Solid Edge part; units mm, degrees
sketch "Sketch1" plane through (0, 0, 0) normal (0, 0, 1) x (1, 0, 0)
  line L0 (0, 0) -> (-248.03, 0)
  line L1 (-248.03, 0) -> (-248.03, -85)
  line L2 (-248.03, -85) -> (0, -85)
  line L3 (0, -85) -> (0, 0)
extrude "Protrusion1" add sketch "Sketch1" against normal blind 20.4
sketch "Sketch2" plane through (-124.015, -42.5, 0) normal (0, 0, 1) x (1, 0, 0)
  circle A0 centre (155, -6) radius 55
  circle A1 centre (57.5, -9) radius 6.7
extrude "ExtrudedCutout_1" cut sketch "Sketch2" against normal blind 20.5
chamfer "Chamfer_2" distance 2 angle 45 1 edges at (-10.158, -85, -10.2)
fillet "Round_1" radius 1 1 edges at (0, 0, -10.2)
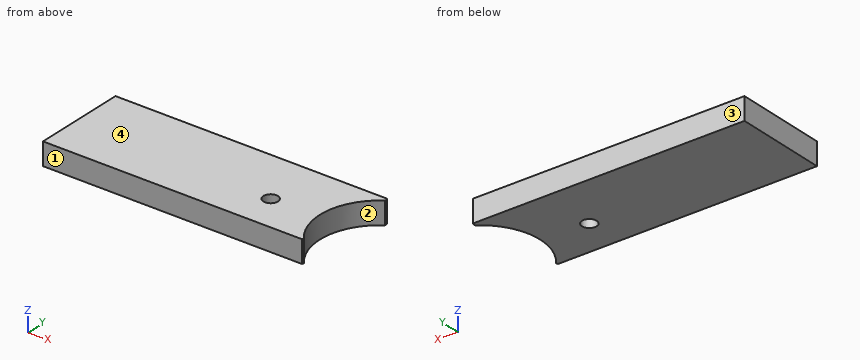
Design review of the part built by this model. Coordinates are the model's own, in mm. Face numbers are marked on the shaded views. Coordinates: 2 decimals unless noted, no trailing zeros. Order: outer loops, then holes, each group sorted by start corner. A loop starts at its lowest first (then second) coordinate and runs counter-clockwise, first axis right, second up. Notation, with made-up numbers: (-34, 14.25) -> (-8, 14.25) arc R21 cw to (-8, 53.25) -> close; hole circle Ø8 at (86.5, 24.5). An arc over 180 degrees is marked (long way). Use one line per item in the form item = value. Start each with the question number.
(1) Insertion check: pin 1 (8 mm diameter, centred on x = -66.515, y = -51.5, fed in from -Z). The pin has a flat end and moves straight along its axis. Give the tip position at first contact, or say it passes through.
(2) Add section D-D on y = -70.5. State the section outline as (x, z) points.
(3) Add section C-C on x = -63. State the section outline as (y, z) points, plus the area to 3 significant figures.
(4) Add section B-B on y = -51.5. State the section outline as (x, z) points (3 decimals), plus the area to 3 significant figures.
(5) The part is to be moulded in two halves that separate along Y. For the marked faces 1, 2, 3 and 4, say which applies: +Y half, -Y half, draft (parallel to the pull), parting line (faces both ways), or undercut.
(6) Add section A-A on z = -5.25. State the section outline as (x, y) points (1 decimal), plus the area to 3 significant figures.
(7) For probe 1 along X at (y, z) = (-68, -3.5); probe 2 along X at (y, z) = (-46.5, -17); probe 3 along X at (y, z) = (-55.5, -17.25), list the stretches that pass through material, from the lowest coordinate up.
Answer block:
q1.pin_1 = through
q2.outline = (-248.03, -20.4) -> (-19.42, -20.4) -> (-19.42, 0) -> (-248.03, 0) -> close
q3.outline = (-85, -20.4) -> (-57.2, -20.4) -> (-57.2, 0) -> (-85, 0) -> close; (-45.8, -20.4) -> (0, -20.4) -> (0, 0) -> (-45.8, 0) -> close
q3.area = 1,500 mm²
q4.outline = (-248.03, -20.4) -> (-73.215, -20.4) -> (-73.215, 0) -> (-248.03, 0) -> close; (-59.815, -20.4) -> (-23.933, -20.4) -> (-23.933, 0) -> (-59.815, 0) -> close
q4.area = 4,300 mm²
q5.face_1 = -Y half
q5.face_2 = undercut
q5.face_3 = +Y half
q5.face_4 = draft
q6.outline = (-248, -85) -> (-12.1, -85) -> (-11.4, -83.5) arc R55 cw to (0, -3.1) -> (0, -1) arc R1 ccw to (-1, 0) -> (-248, 0) -> close; hole circle Ø13.4 at (-66.5, -51.5)
q6.area = 19,500 mm²
q7.probe_1 = -248.03 to -20.44
q7.probe_2 = -248.03 to -70.97, -62.06 to -23.98
q7.probe_3 = -248.03 to -71.89, -61.14 to -23.57
